from build123d import *

# Parameters (mm, degrees)
SKETCH1_W            = 60
SKETCH1_H            = 60
SKETCH1_R            = 27.5
BOSS_EXTRUDE2_DEPTH  = 2
BOSS_EXTRUDE3_DEPTH  = 1
BOSS_EXTRUDE4_DEPTH  = 59
BOSS_EXTRUDE5_DEPTH  = 20
SKETCH6_W            = 4
SKETCH6_H            = 14.848240743
CUT_EXTRUDE1_DEPTH   = 20
BOSS_EXTRUDE6_DEPTH  = 2
SKETCH9_W            = 21
SKETCH9_H            = 33.426406871
BOSS_EXTRUDE8_DEPTH  = 2
SKETCH11_W           = 57.719066806
SKETCH11_H           = 59.906444101
BOSS_EXTRUDE9_DEPTH  = 1.5
CUT_EXTRUDE3_DEPTH   = 44.570078861
BOSS_EXTRUDE10_REACH = 41.922
CUT_EXTRUDE4_DEPTH   = 26.5
SKETCH15_W           = 98.795654727
SKETCH15_H           = 69.251879537
CUT_EXTRUDE5_DEPTH   = 59.5
SKETCH16_R           = 67.668555037
CUT_EXTRUDE6_DEPTH   = 1093.5
SKETCH17_R           = 80.414803425
CUT_EXTRUDE7_DEPTH   = 212.5
SKETCH18_W           = 81.243812254
SKETCH18_H           = 75.888975698
SKETCH18_R           = 27.5
BOSS_EXTRUDE12_DEPTH = 3
BOSS_EXTRUDE13_DEPTH = 2
SKETCH20_R           = 82.636183776
CUT_EXTRUDE8_DEPTH   = 100
SKETCH21_R           = 85.046347758
CUT_EXTRUDE9_DEPTH   = 22
SKETCH23_R           = 93.159906211
CUT_EXTRUDE11_DEPTH  = 94
SKETCH24_R           = 86.281354965
CUT_EXTRUDE12_DEPTH  = 48
SKETCH25_R           = 66.198443884
CUT_EXTRUDE13_DEPTH  = 170
BOSS_EXTRUDE14_DEPTH = 2
SKETCH27_W           = 18.5
SKETCH27_H           = 15.5
SKETCH27_W_2         = 16
SKETCH27_H_2         = 12
BOSS_EXTRUDE15_DEPTH = 5


with BuildPart() as part:
    # Sketch1 → Boss-Extrude2 (new body)
    with BuildSketch(Plane.XY):
        with Locations((28, 28)):
            Rectangle(SKETCH1_W, SKETCH1_H)
        with Locations((28, 28)):
            Circle(SKETCH1_R, mode=Mode.SUBTRACT)
    extrude(amount=BOSS_EXTRUDE2_DEPTH)

    # Sketch2 → Boss-Extrude3 (add)
    with BuildSketch(Plane.ZY.offset(2)):
        Polygon((2, 58), (-1.535533906, 61.535533906), (-32.535533906, 30.535533906), (0, -2), (0, 58), align=None)
    extrude(amount=-BOSS_EXTRUDE3_DEPTH)

    # Sketch3 → Boss-Extrude4 (add)
    with BuildSketch(Plane(origin=(-1, 0, 0), x_dir=(0, 0, -1), z_dir=(1, 0, 0))):
        Polygon((0, 58), (2.535533906, 60.535533906), (1.535533906, 61.535533906), (-2, 58), align=None)
    extrude(amount=BOSS_EXTRUDE4_DEPTH)

    # Sketch5 → Boss-Extrude5 (add)
    with BuildSketch(Plane(origin=(-1, 0, 0), x_dir=(0, 0, -1), z_dir=(1, 0, 0))):
        Polygon((2.535533906, 60.535533906), (32.535533906, 30.535533906), (31.121320344, 29.121320344), (1.121320344, 59.121320344), align=None)
    extrude(amount=BOSS_EXTRUDE5_DEPTH)

    # Sketch6 → Cut-Extrude1 (cut)
    with BuildSketch(Plane(origin=(0, 31.535533906, -31.535533906), x_dir=(1, 0, 0), z_dir=(0, 0.707106781, -0.707106781))):
        with Locations((2.5, -8.692828461)):
            Rectangle(SKETCH6_W, SKETCH6_H)
    extrude(amount=-CUT_EXTRUDE1_DEPTH, mode=Mode.SUBTRACT)

    # Sketch7 → Boss-Extrude6 (add)
    with BuildSketch(Plane(origin=(0, 31.535533906, -31.535533906), x_dir=(1, 0, 0), z_dir=(0, 0.707106781, -0.707106781))):
        Polygon((19, 1.414213562), (58, -41.012193309), (19, -41.012193309), align=None)
    extrude(amount=-BOSS_EXTRUDE6_DEPTH)

    # Sketch9 → Boss-Extrude8 (add)
    with BuildSketch(Plane(origin=(0, -1, -1), x_dir=(-1, 0, 0), z_dir=(0, -0.707106781, -0.707106781))):
        with Locations((-8.5, 13.884776311)):
            Rectangle(SKETCH9_W, SKETCH9_H)
    extrude(amount=-BOSS_EXTRUDE8_DEPTH)

    # Sketch11 → Boss-Extrude9 (add)
    with BuildSketch(Plane(origin=(22.469349188, -2.1452201, -27.064933845), x_dir=(-0.676752968, -0.520579206, -0.520579206), z_dir=(0.637576713, -0.060871473, -0.767978254))):
        with Locations((-40.536850198, 1.112103584)):
            Rectangle(SKETCH11_W, SKETCH11_H)
    extrude(amount=-BOSS_EXTRUDE9_DEPTH)

    # Sketch12 → Cut-Extrude3 (cut, through all)
    with BuildSketch(Plane(origin=(21.512984119, -2.053912891, -25.912966464), x_dir=(0.770386874, 0.050377589, 0.635583325), z_dir=(-0.637576713, 0.060871473, 0.767978254))):
        Polygon((43.649580839, -2.15177531), (42.724580914, -9.59239755), (74.742668884, 7.823146391), (47.317707346, 58.243324712), align=None)
    extrude(amount=-CUT_EXTRUDE3_DEPTH, mode=Mode.SUBTRACT)

    # Boss-Extrude10: up to this face of the body (flat: up to its plane)
    boss_extrude10_end = Plane(part.part.faces().sort_by_distance((41.682824106, 19.529388287, -10.878669739))[0])
    # Sketch13 → Boss-Extrude10 (add, up to the picked face)
    with BuildSketch(Plane(origin=(19, 0, 0), x_dir=(0, 0, -1), z_dir=(1, 0, 0)), mode=Mode.PRIVATE) as boss_extrude10_sk1:
        Polygon((21.221825407, 22.050252532), (22.636038969, 20.636038969), (-1, -3), (-2.414213562, -1.585786438), align=None)
    boss_extrude10_tool1 = split(extrude(boss_extrude10_sk1.sketch, amount=BOSS_EXTRUDE10_REACH, mode=Mode.PRIVATE), bisect_by=boss_extrude10_end, keep=Keep.BOTH, mode=Mode.PRIVATE)
    add(boss_extrude10_tool1.solids().sort_by_distance((19, 9.525126, -10.110913))[0])

    # Sketch14 → Cut-Extrude4 (cut)
    with BuildSketch(Plane(origin=(21.512984119, -2.053912891, -25.912966464), x_dir=(0.770386874, 0.050377589, 0.635583325), z_dir=(-0.637576713, 0.060871473, 0.767978254))):
        Polygon((41.962116988, -3.069634642), (7.93553086, 22.360087902), (-27.775626078, 49.048772133), (11.868884468, -40.106499749), (63.912471384, -11.732484985), align=None)
    extrude(amount=-CUT_EXTRUDE4_DEPTH, mode=Mode.SUBTRACT)

    # Sketch15 → Cut-Extrude5 (cut)
    with BuildSketch(Plane(origin=(0, -1, -1), x_dir=(-1, 0, 0), z_dir=(0, -0.707106781, -0.707106781))):
        with Locations((-41.379570233, 23.483837132)):
            Rectangle(SKETCH15_W, SKETCH15_H)
    extrude(amount=CUT_EXTRUDE5_DEPTH, mode=Mode.SUBTRACT)

    # Sketch16 → Cut-Extrude6 (cut)
    with BuildSketch(Plane(origin=(22.469349188, -2.1452201, -27.064933845), x_dir=(-0.770386874, -0.050377589, -0.635583325), z_dir=(0.637576713, -0.060871473, -0.767978254))):
        with Locations((-31.476014369, 28.909090329)):
            Circle(SKETCH16_R)
    extrude(amount=CUT_EXTRUDE6_DEPTH, mode=Mode.SUBTRACT)

    # Sketch17 → Cut-Extrude7 (cut)
    with BuildSketch(Plane(origin=(58, 0, 0), x_dir=(0, 0, -1), z_dir=(1, 0, 0))):
        with Locations((-1.230106157, 56.933870915)):
            Circle(SKETCH17_R)
    extrude(amount=CUT_EXTRUDE7_DEPTH, mode=Mode.SUBTRACT)

    # Sketch18 → Boss-Extrude12 (add)
    with BuildSketch(Plane.XY.offset(2)):
        with Locations((28, 28)):
            Rectangle(SKETCH18_W, SKETCH18_H)
        with Locations((28, 28)):
            Circle(SKETCH18_R, mode=Mode.SUBTRACT)
    extrude(amount=-BOSS_EXTRUDE12_DEPTH)

    # Sketch19 → Boss-Extrude13 (add)
    with BuildSketch(Plane(origin=(22.469349188, -2.1452201, -27.064933845), x_dir=(-0.770386874, -0.050377589, -0.635583325), z_dir=(0.637576713, -0.060871473, -0.767978254))):
        Polygon((-48.688581729, 61.770152877), (-46.120529867, 41.112957892), (-46.120529867, 60.372277801), align=None)
        Polygon((-46.120529867, 41.112957892), (-40.895361663, -0.917859332), (4.352561758, 32.898114271), (-46.120529867, 60.372277801), align=None)
    extrude(amount=-BOSS_EXTRUDE13_DEPTH)

    # Sketch20 → Cut-Extrude8 (cut)
    with BuildSketch(Plane(origin=(22.469349188, -2.1452201, -27.064933845), x_dir=(-0.770386874, -0.050377589, -0.635583325), z_dir=(0.637576713, -0.060871473, -0.767978254))):
        with Locations((-26.945010232, 29.388055989)):
            Circle(SKETCH20_R)
    extrude(amount=CUT_EXTRUDE8_DEPTH, mode=Mode.SUBTRACT)

    # Sketch21 → Cut-Extrude9 (cut)
    with BuildSketch(Plane(origin=(0, 31.535533906, -31.535533906), x_dir=(1, 0, 0), z_dir=(0, 0.707106781, -0.707106781))):
        with Locations((19.590538608, -26.723706738)):
            Circle(SKETCH21_R)
    extrude(amount=CUT_EXTRUDE9_DEPTH, mode=Mode.SUBTRACT)

    # Sketch23 → Cut-Extrude11 (cut)
    with BuildSketch(Plane.ZY.offset(2)):
        with Locations((-13.361611356, 29.287919071)):
            Circle(SKETCH23_R)
    extrude(amount=CUT_EXTRUDE11_DEPTH, mode=Mode.SUBTRACT)

    # Sketch24 → Cut-Extrude12 (cut)
    with BuildSketch(Plane(origin=(0, -1, -1), x_dir=(-1, 0, 0), z_dir=(0, -0.707106781, -0.707106781))):
        with Locations((-12.739775939, 17.868647739)):
            Circle(SKETCH24_R)
    extrude(amount=CUT_EXTRUDE12_DEPTH, mode=Mode.SUBTRACT)

    # Sketch25 → Cut-Extrude13 (cut)
    with BuildSketch(Plane.XY.offset(2)):
        with Locations((30.355803371, 29.212907652)):
            Circle(SKETCH25_R)
    extrude(amount=CUT_EXTRUDE13_DEPTH, mode=Mode.SUBTRACT)

    # Sketch26 → Boss-Extrude14 (add)
    with BuildSketch(Plane(origin=(0, -1, -1), x_dir=(-1, 0, 0), z_dir=(0, -0.707106781, -0.707106781))):
        Polygon((-15, 30.597979746), (-15, 44.597979746), (-18.325381464, 44.597979746), (-30.150830661, 29.463089368), (-15, 29.463089368), align=None)
    extrude(amount=-BOSS_EXTRUDE14_DEPTH)

    # Sketch27 → Boss-Extrude15 (add)
    with BuildSketch(Plane(origin=(0, -1, -1), x_dir=(-1, 0, 0), z_dir=(0, -0.707106781, -0.707106781))):
        with Locations((-7.25, 36.847979746)):
            Rectangle(SKETCH27_W, SKETCH27_H)
        with Locations((-7, 36.597979746)):
            Rectangle(SKETCH27_W_2, SKETCH27_H_2, mode=Mode.SUBTRACT)
    extrude(amount=BOSS_EXTRUDE15_DEPTH)


solid = part.part
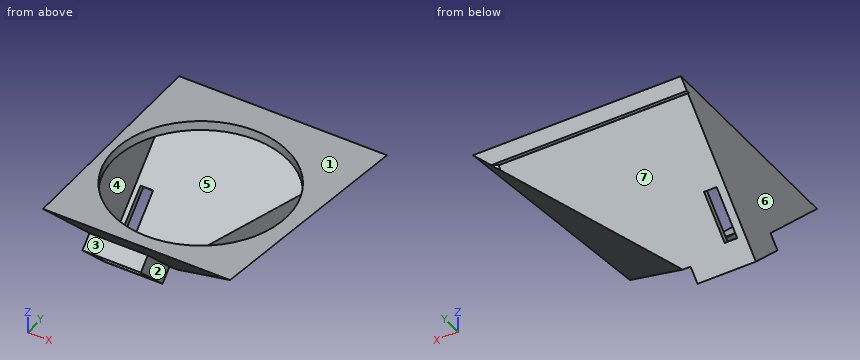
Can you work these out from the model? Positions are in its coordinate system, mm. Face numbers are marked on the shaded views. A direction names the side the tool comes from. Give positions to 0.01 mm unless a question says otherwise; leave off trailing zeros. Order: outer loops, then holes, each group sorted by start corner. A loop starts at its lowest first (then second) coordinate and runs counter-clockwise, first axis right, second up. Notation, with made-up numbers: (51, -37.75) - (67, -37.75) arc R27 ccw to (67, -17.75) - close; hole circle Ø4 at (10.25, 58.25). An arc over 180 degrees is marked (long way). Write each question's results on one line, items separated by ' | '.
1) Please list where these lines run through material, in increasing order: line 1 along Z through (x, y) = (1.5, 41); line 2 along X through (y, z) = (17, -11.5); line 3 along X through (y, z) = (28, 0). Write a range as [from, to].
Final values:
line 1: z = [-1, 2] | line 2: x = [-2, -1], [39.91, 43.05] | line 3: x = [-2, 0.5], [54.81, 57.95]
2) Suppose I cut it at B-B, the plane y = 33.5. Write out the boundary of the cut face in (x, z).
Final values:
outline: (-2, -29.57) - (0.5, -29.57) - (0.5, -26.74) - (-1, -26.74) - (-1, -1) - (1.06, -1) - (1.06, 2) - (-2, 2) - close; (4.5, -29.57) - (22.85, -29.57) - (22.94, -29.43) - (22.98, -29.47) - (60.88, 2) - (54.94, 2) - (54.94, -0.33) - (23.12, -26.74) - (4.5, -26.74) - close
3) I'm going to push flat-ended pins straight in: pin 1 Ø8 at (y, z) = (18, -11.5) entering from +X; pin 2 Ø10 at (y, z) = (22.5, -22.5) entering from +X; pin 3 Ø10 at (y, z) = (28, -26) entering from +X; pin 4 Ø12 at (x, z) = (37, -27) entering from -Y. Where does each tip first touch, or does it pass through?
Final values:
pin 1: stops at x = 47.97 | pin 2: stops at x = 36.36 | pin 3: stops at x = 32.67 | pin 4: passes through
4) On a 3-axis mill with a long thin cutter (end or side, diameter ignored), from which of +Z, -Z, +X, -X, +Y, -Y can I reach the whole of each face in a straight line? I mean the marked faces 1, 2 and 3. Say none if no direction works.
Final values:
face 1: +Z, +X, -X, +Y, -Y | face 2: -Z, +X, -Y | face 3: +X, -X, -Y
5) Suppose I cut it at C-C, the plane z = -27. Write out the boundary of the cut face in (x, y), then the cut area to 3 significant figures.
Final values:
outline: (-2, 17.93) - (-1, 17.93) - (-1, 33.24) - (0.5, 33.24) - (0.5, 36.07) - (-2, 36.07) - close; (4.5, 33.24) - (22.79, 33.24) - (22.27, 27.83) - (15, 27.83) - (15, 17.93) - (16.5, 17.93) - (16.5, 25) - (25.14, 25) - (26.19, 35.97) - (26.11, 35.93) - (26.2, 36.07) - (4.5, 36.07) - close | area: 140 mm^2
6) If we mould it in two halves opening along X, with no side actions, what happens to the marked faces 4, 5, 6 and 7? For each: pulls with the +X half, pulls with the -X half, needs draft (parallel to the pull), parting line crosses it, or undercut.
Final values:
face 4: undercut | face 5: undercut | face 6: pulls with the -X half | face 7: needs draft
7) Suppose I cut it at A-A, the plane x = 9.5. Write out the boundary of the cut face in (y, z).
Final values:
outline: (-4, 2) - (19.58, -21.58) - (16.04, -25.11) - (17.1, -26.17) - (22.05, -21.22) - (1.83, -1) - (7.65, -1) - (7.65, 2) - close; (25.59, -34.66) - (27, -36.07) - (61.54, -1.54) - (61, -1) - (62.07, -1) - (65.07, 2) - (48.35, 2) - (48.35, -1) - (59, -1) - (59.12, -1.12) - close
8) Suppose I cut it at D-D, the plane x = 42.5. Write out the boundary of the cut face in (y, z).
Final values:
outline: (-4, 2) - (9.35, -11.35) - (48.52, -14.45) - (48.54, -14.39) - (48.61, -14.46) - (61.54, -1.54) - (61, -1) - (62.07, -1) - (65.07, 2) - (51.37, 2) - (51.37, -1) - (59, -1) - (59.12, -1.12) - (48.4, -11.84) - (9.59, -8.76) - (1.83, -1) - (4.63, -1) - (4.63, 2) - close
